Check sheet for the drawn part. Datum: minimum x, y, z corner. Units: mm. Coordinates: 2 decimals unless noted, no trailing zeros. Write each loop counter-clockwise with the first axis right and the second up, starting at its lowest first coordinate (ties: lowest second). Pieces come first, ordered by that corner, then holes. Notation, with made-up numbers: (-23.75, 35) - (32.25, 35) arc R21 ccw to (32.25, 58) - close; hole circle Ø4 at (57.25, 32.25). An arc over 180 degrees is marked (long way). Answer as CSV lines item,"result". Start each with the question number.
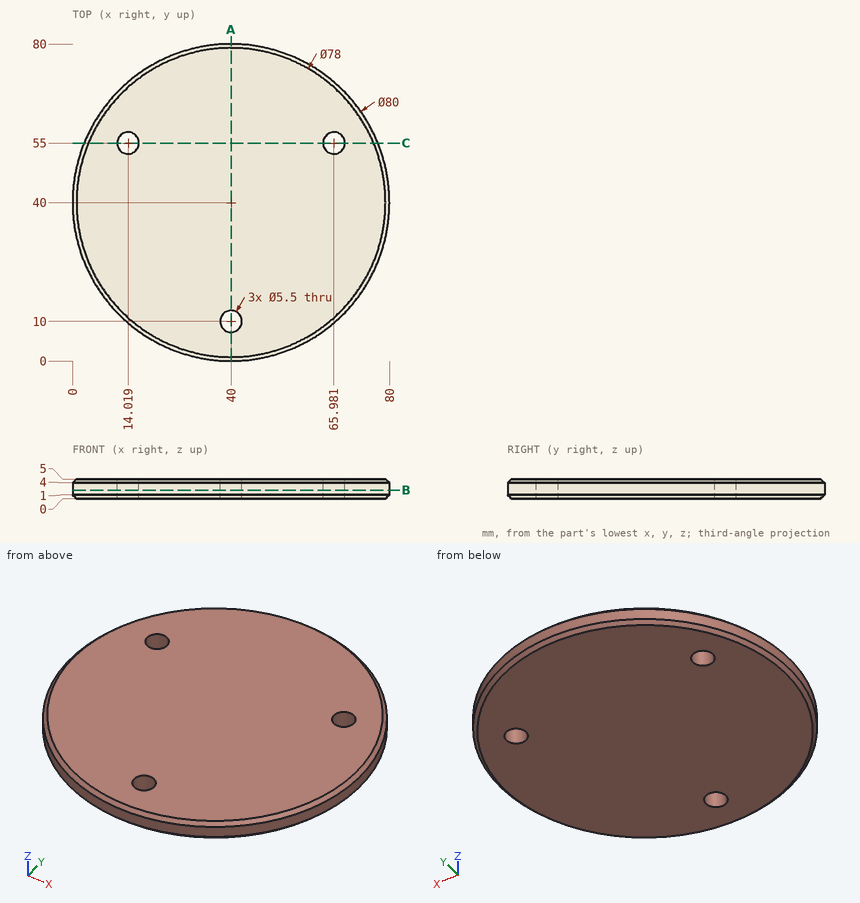
(1) Cross-section at A-A on x = 40. Record the boundary of the cut face in (y, z).
(2) Material ranges on probe 1 along X at (y, z) = (54, 1.35); probe 2 along Y at (x, z) = (39, 1.1); probe 3 along X at (y, z) = (10, 2), recorded low to high. Write a range as from..to.
(3) Go/stop test with a flat-tipped pin: P1, Ø2, axis at y = 67.5, z = 1, coming from the -X side. Record where the tip stops, or that it passes through.
(4) Cross-section at C-C on y = 55. State how many separate pieces and enclosed holes the cut face has, plus the area to 3 significant figures.
(5) Cross-section at B-B on z = 2.2. Record the boundary of the cut face in (x, y), plus the area to 3 significant figures.
Checked values:
1,outline,"(0, 1) - (1, 0) - (7.25, 0) - (7.25, 5) - (1, 5) - (0, 4) - close; (12.75, 0) - (79, 0) - (80, 1) - (80, 4) - (79, 5) - (12.75, 5) - close"
2,probe 1,"2.53..11.46, 16.58..63.42, 68.54..77.47"
2,probe 2,"0.01..7.44, 12.56..79.99"
2,probe 3,"13.54..37.25, 42.75..66.46"
3,P1,"x = 10.04"
4,separate pieces,"3"
4,enclosed holes,"0"
4,area,"314 mm^2"
5,outline,"circle Ø80 at (40, 40); hole circle Ø5.5 at (14.02, 55); hole circle Ø5.5 at (40, 10); hole circle Ø5.5 at (65.98, 55)"
5,area,"4,960 mm^2"
